Drawing for the job (mm, zero at the part's lowest x, y, z). Round coordinates to 2 decimals unless told otherwise and drop trailing zeros. Loops run counter-clockwise (first coordinate to the right, second up) from the corner with the lowest first, then second, coordinate; pieces in that order, holes last. Notation, with made-up numbers: M -35,26 L 20,26 A23 ccw 20,40 Z; hole C 69,53.25 d3. An arc over 180 degrees is marked long. Answer in a Markdown table with one row per item.
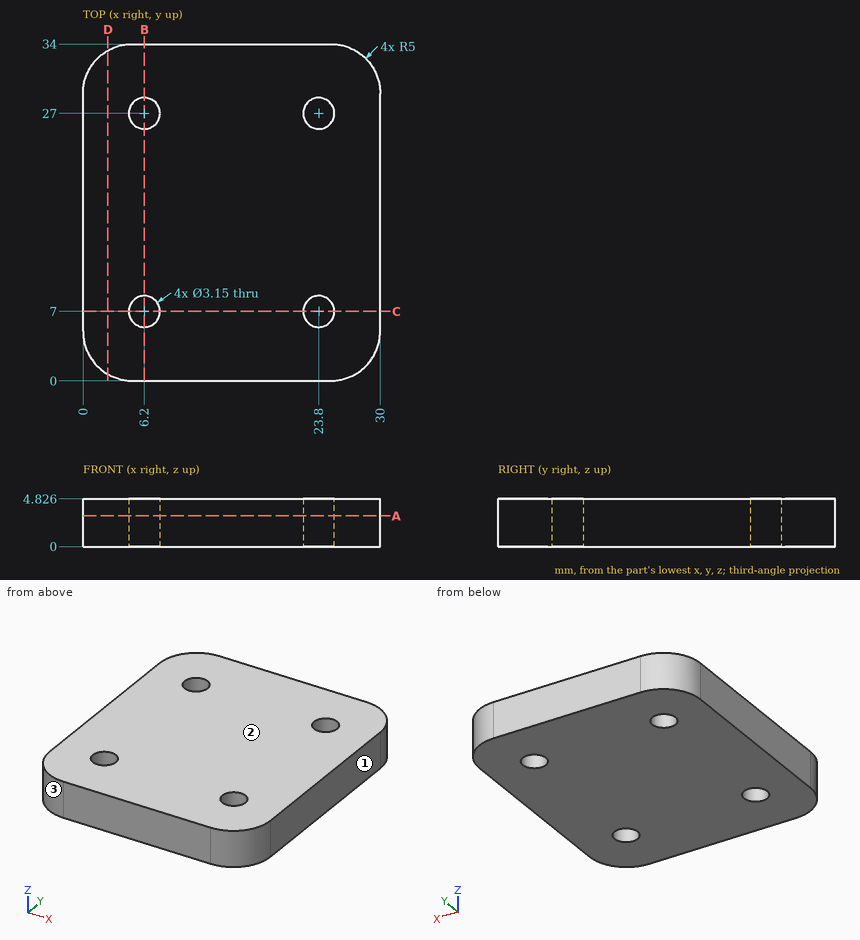
1. Mould opens along X. For the marked faces 1, 2 and 3 say: +X half, -X half, draft (parallel to the pull), parting line (faces both ways), or undercut.
Verdict:
| item | result |
|---|---|
| face 1 | +X half |
| face 2 | draft |
| face 3 | -X half |
2. Saw through at A-A (z = 3.1). Write the cut outline in (x, y) (3 decimals), and give its area (3 significant figures).
Verdict:
| item | result |
|---|---|
| outline | M 0,5 A5 ccw 5,0 L 25,0 A5 ccw 30,5 L 30,29 A5 ccw 25,34 L 5,34 A5 ccw 0,29 Z; hole C 6.2,7 d3.15; hole C 6.2,27 d3.15; hole C 23.8,7 d3.15; hole C 23.8,27 d3.15 |
| area | 967 mm² |
3. Saw through at D-D (x = 2.5). Write the cut outline in (y, z), and give its area (3 significant figures).
Verdict:
| item | result |
|---|---|
| outline | M 0.67,0 L 33.33,0 L 33.33,4.83 L 0.67,4.83 Z |
| area | 158 mm² |
4. Wall check: probe 1 along Y at (x, z) = (6.2, 3.2) (3 decimals); probe 2 along Y at (x, z) = (5, 2.65); probe 3 along X at (y, z) = (26.5, 3.7). Give the ranges that are in metal, low to high.
Verdict:
| item | result |
|---|---|
| probe 1 | y = 0 to 5.425, 8.575 to 25.425, 28.575 to 34 |
| probe 2 | y = 0 to 5.98, 8.02 to 25.98, 28.02 to 34 |
| probe 3 | x = 0 to 4.71, 7.69 to 22.31, 25.29 to 30 |
5. Saw through at C-C (y = 7). Write the cut outline in (x, z) (3 decimals).
Verdict:
| item | result |
|---|---|
| outline | M 0,0 L 4.625,0 L 4.625,4.826 L 0,4.826 Z; M 7.775,0 L 22.225,0 L 22.225,4.826 L 7.775,4.826 Z; M 25.375,0 L 30,0 L 30,4.826 L 25.375,4.826 Z |
6. Saw through at B-B (x = 6.2). Write the cut outline in (y, z) (3 decimals), and give its area (3 significant figures).
Verdict:
| item | result |
|---|---|
| outline | M 0,0 L 5.425,0 L 5.425,4.826 L 0,4.826 Z; M 8.575,0 L 25.425,0 L 25.425,4.826 L 8.575,4.826 Z; M 28.575,0 L 34,0 L 34,4.826 L 28.575,4.826 Z |
| area | 134 mm² |
